```python
from build123d import *

# Parameters (mm, degrees)
SKETCH1_R           = 17
SKETCH1_R_2         = 12
BOSS_EXTRUDE1_DEPTH = 80
CHAMFER1_SIZE       = 2
CHAMFER1_SIZE2      = 22.860104606
BOSS_EXTRUDE2_START = 5
SKETCH2_R           = 17
BOSS_EXTRUDE2_DEPTH = 5
SKETCH3_R           = 9
SKETCH3_R_2         = 4
BOSS_EXTRUDE3_DEPTH = 3
BOSS_EXTRUDE4_START = 3
SKETCH3_3_R         = 4
BOSS_EXTRUDE4_DEPTH = 7
FILLET1_R           = 12
CHAMFER2_SIZE       = 0.5


with BuildPart() as part:
    # Sketch1 → Boss-Extrude1 (new body)
    with BuildSketch(Plane.XY):
        Circle(SKETCH1_R)
        Circle(SKETCH1_R_2, mode=Mode.SUBTRACT)
    extrude(amount=BOSS_EXTRUDE1_DEPTH)

    # Chamfer1
    chamfer1_edges = [part.edges().sort_by_distance(p)[0] for p in [
        (-12, 0, 80),
    ]]
    chamfer1_side = [part.faces().sort_by_distance(p)[0] for p in [
        (-16.519167389, 0, 80),
    ]]
    chamfer(chamfer1_edges, length=CHAMFER1_SIZE, length2=CHAMFER1_SIZE2, reference=chamfer1_side[0])

    # Sketch2 → Boss-Extrude2 (add)
    with BuildSketch(Plane(origin=(0, 0, 0), x_dir=(-1, 0, 0), z_dir=(0, 0, -1)).offset(BOSS_EXTRUDE2_START)):
        Circle(SKETCH2_R)
    extrude(amount=-BOSS_EXTRUDE2_DEPTH)

    # Sketch3 → Boss-Extrude3 (add)
    # profile 1 of 2: a face of its own
    with BuildSketch(Plane(origin=(0, 0, -5), x_dir=(-1, 0, 0), z_dir=(0, 0, -1))):
        Circle(SKETCH3_R)
        Circle(SKETCH3_R_2, mode=Mode.SUBTRACT)
    # profile 2 of 2: a face of its own
    with BuildSketch(Plane(origin=(0, 0, -5), x_dir=(-1, 0, 0), z_dir=(0, 0, -1))):
        Circle(SKETCH3_R_2)
    extrude(amount=BOSS_EXTRUDE3_DEPTH)

    # Sketch3<3> → Boss-Extrude4 (add)
    with BuildSketch(Plane(origin=(0, 0, -5), x_dir=(-1, 0, 0), z_dir=(0, 0, -1)).offset(BOSS_EXTRUDE4_START)):
        Circle(SKETCH3_3_R)
    extrude(amount=BOSS_EXTRUDE4_DEPTH)

    # Fillet1
    # the kernel refuses this fillet: 12 mm, written as the material it adds along each edge
    with BuildSketch(Plane(origin=(0, 0, -5), x_dir=(-1, 0, 0), z_dir=(0, -1, 0))) as fillet1_piece_1:
        with BuildLine():
            CenterArc((16.937253933, 12), FILLET1_R, 228.590377891, 41.409622109)
            Line((9, 3), (9, 0))
            Line((9, 0), (16.937253933, 0))
        make_face()
    revolve(axis=Axis((0, 0, -5), (0, 0, -1)))

    # Chamfer2
    chamfer2_edges = [part.edges().sort_by_distance(p)[0] for p in [
        (4, 0, -15),
    ]]
    chamfer(chamfer2_edges, length=CHAMFER2_SIZE)


solid = part.part
```
The listing builds one solid part. Answer for the finished solid, in the listing's coordinates (mm). A direction names the side the tool comes from. Coordinates: 2 decimals unless noted, no trailing zeros. Loops run counter-clockwise (first coordinate to the right, second up) from the corner with the lowest first, then second, coordinate; pieces in that order, holes last. Notation, with made-up numbers: M 73.25,74.25 L 86.25,74.25 A25 cw 86.25,101.25 Z; hole C 43,-1 d1. An arc over 180 degrees is marked long. Answer as CSV lines item,"result". Start each with the question number.
(1) Find the intervals of material crossed by L1, parallel to Y at x = 0, z = 40; L2, parallel to Y at x = -6.5, z = 72.5; L3, parallel to X at y = 3, z = 34, in increasing order. Write a range as [from, to].
(2) For faces 5 (the flat face through (0, 0, 0)), 6 (the flat face through (-6, 13, 80)), 7 (the flat face through (-4, -2, -8)), determine the directions among +Z, -Z, +X, -X, +Y, -Y from which every point of the face is accessible in a straight line to the end or side of a thin tool.
(3) The part is cut by section A-A (z = 53). Give the vertices of the cut face in (x, y).
(4) The mould has two halves that part along X. Classify faces 1 (the conical face through (-12.973, 0.571, 68.41)), 2 (the cylindrical face through (0.867, -3.905, -11.204)), 3 (the flat face through (0, 0, -15)), 4 (the cylindrical face through (-11.99, 0.53, 28.17)): pulls with the +X half, pulls with the -X half, needs draft (parallel to the pull), parting line crosses it, or undercut.
(5) Given pin 1 (2 mm diameter, centred on x = -2, z = 17.5, fed in from -Y); pin 2 (7 mm diameter, centred on x = -1.5, y = -1.5, fed in from +Z); pin 3 (3 mm diameter, centred on x = 7, y = -8.5, fed in from -Z), each flat-ended and moving along its own axis, determine where each tip first touches the part or whether it passes through.
(6) The part is cut by section B-B (x = 0). Give the vertices of the cut face in (y, z).
(7) The part is cut by section C-C (z = 65.5). Give the vertices of the cut face in (x, y), and give its area (3 significant figures).
Determined:
1,L1,"[-17, -12], [12, 17]"
1,L2,"[-15.71, -11.65], [11.65, 15.71]"
1,L3,"[-16.73, -11.62], [11.62, 16.73]"
2,face 5,"+Z"
2,face 6,"+Z, +X, -X, +Y, -Y"
2,face 7,"-Z"
3,outline,"C 0,0 d34; hole C 0,0 d24"
4,face 1,"undercut"
4,face 2,"parting line crosses it"
4,face 3,"needs draft"
4,face 4,"undercut"
5,pin 1,"y = -16.97"
5,pin 2,"z = 0"
5,pin 3,"z = -7.57"
6,outline,"M -17,-5 L -16.94,-5 A12 cw -9,-8 L -4,-8 L -4,-14.5 L -3.5,-15 L 3.5,-15 L 4,-14.5 L 4,-8 L 9,-8 A12 cw 16.94,-5 L 17,-5 L 17,80 L 14,80 L 12,57.14 L 12,0 L -12,0 L -12,57.14 L -14,80 L -17,80 Z"
7,outline,"C 0,0 d34; hole C 0,0 d25.46"
7,area,"399 mm2"
